Print and shaded views of the part. All mm, measured from the part's lowest x, y and z. A direction names the side the tool comes from. Give positions to 0.01 mm unless a question says otherwise; leave off trailing zeros. Write each loop counter-clockwise with the first axis right and the second up, starting at its lowest first coordinate (ties: lowest second). Pieces come first, ordered by that corner, then holes. Notation, with made-up numbers: (-6, 7) -> (38, 7) arc R13 cw to (38, 30) -> close; hole circle Ø3 at (62, 89.25). An arc over 180 degrees is marked (long way). Put each result on its own line as item: value.
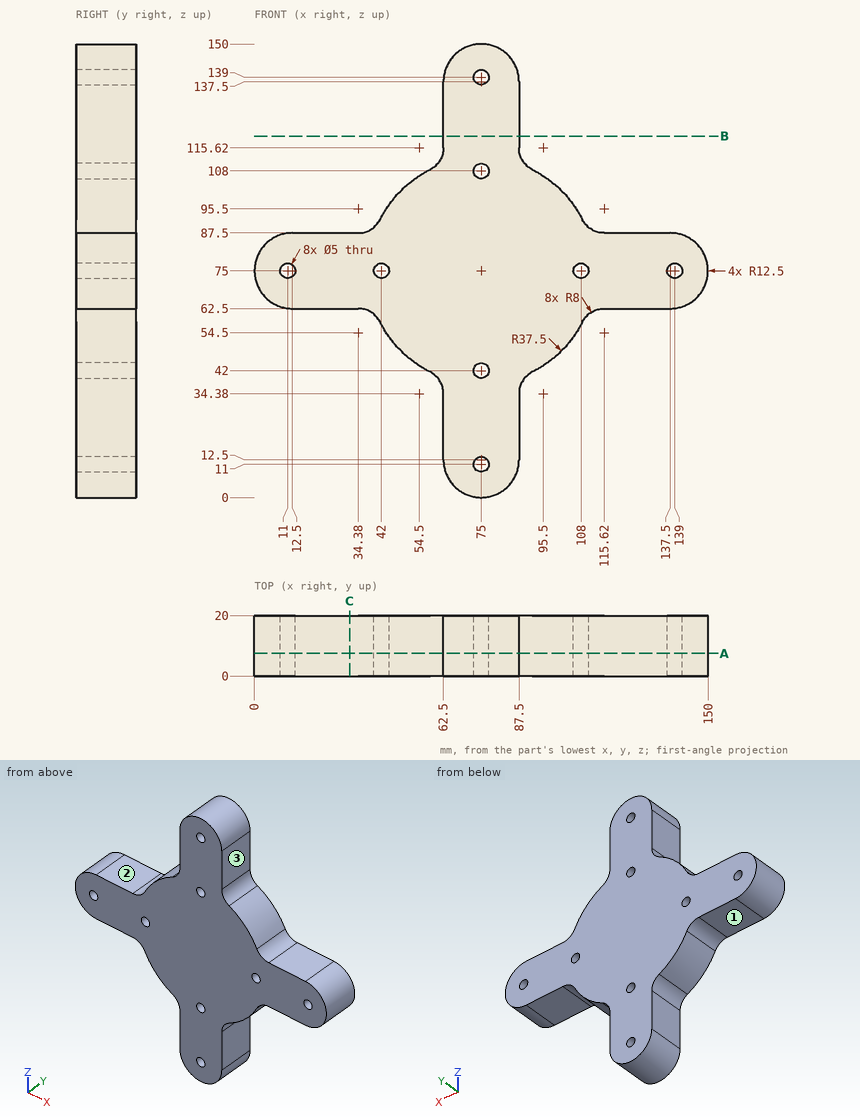
1) Slice it at A-A (y = 7.5). Give the number of separate pieces and of enclosed holes in the cut face, plus the area to 3 significant figures.
Filled sheet:
separate pieces: 1
enclosed holes: 8
area: 7,850 mm2
2) Tool access for the marked faces 1, 2 and 3: list every direction of +Z, -Z, +X, -X, +Y, -Y with a clear straight run to the whole face (end or side of a thin tool).
Filled sheet:
face 1: -Z, -X, +Y, -Y
face 2: +Z, -X, +Y, -Y
face 3: +Z, +X, +Y, -Y
3) Pin check, flat tips, straight feed: pin 1 (10 mm diameter, centred on y = 12, z = 20, fed in from +X); pin 2 (10 mm diameter, centred on y = 7.5, z = 64, fed in from -X); pin 3 (8 mm diameter, centred on y = 9.5, z = 65.5, fed in from +X) (1 decimal). Stop position of each tip, or through.
Filled sheet:
pin 1: x = 87.5
pin 2: x = 1.53
pin 3: x = 148.7
4) Slice it at B-B (z = 119.5). Write the cut outline in (x, y).
Filled sheet:
outline: (62.5, 0) -> (87.5, 0) -> (87.5, 20) -> (62.5, 20) -> close
5) Slice it at C-C (x = 31.5). Write the cut outline in (y, z), plus the area to 3 significant figures.
Filled sheet:
outline: (0, 62.5) -> (20, 62.5) -> (20, 87.5) -> (0, 87.5) -> close
area: 500 mm2
6) Wall check: L1, parallel to X at y = 15.5, z = 11; L2, parallel to X at y = 18, z = 21; L3, parallel to Z at x = 137.5, y = 14.5. Give the ranges that are in metal, low to high.
Filled sheet:
L1: 62.59 to 72.5, 77.5 to 87.41
L2: 62.5 to 87.5
L3: 62.5 to 73, 77 to 87.5
